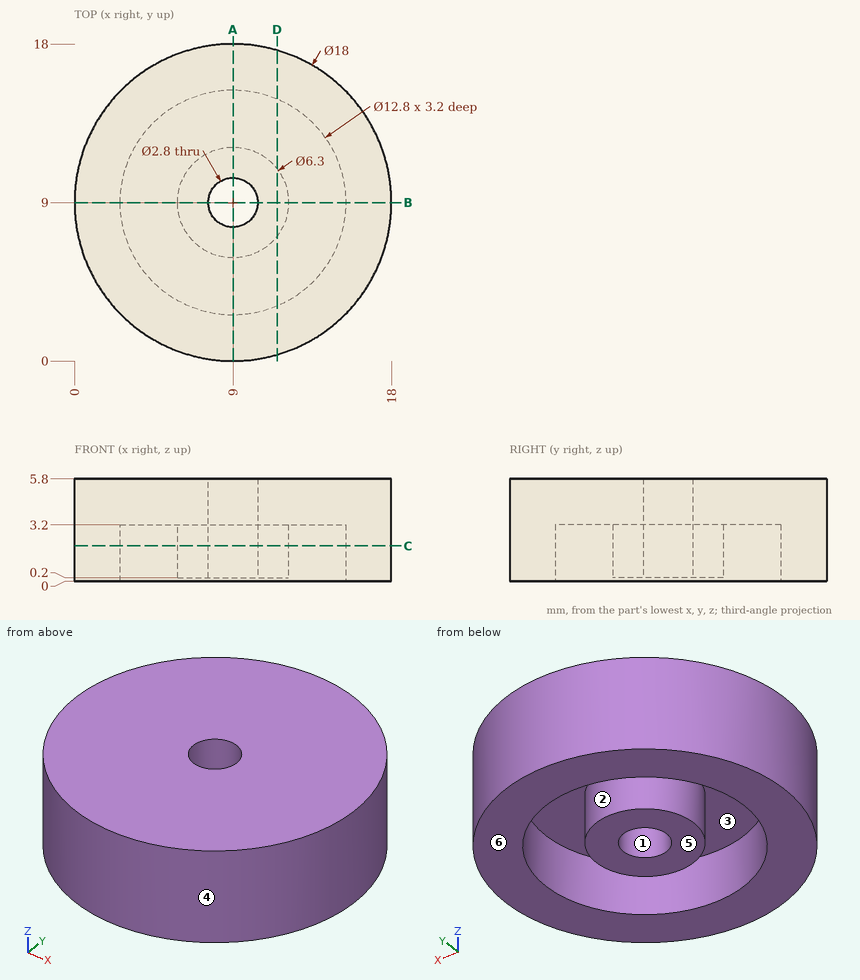
Design review of the part shown in the three views and the two pictorial views. Dimensions are in mm from the part's minimum x, y and z. A direction names the side the tool comes from. Round coordinates to 2 decimals unless told otherwise and drop trailing zeros. Write each loop counter-clockwise with the first axis right and the second up, starting at its lowest first coordinate (ties: lowest second). Pieces come first, ordered by that corner, then holes.
Item 1: Wall thickness on L1, parallel to Y at x = 9, z = 2.6; L2, parallel to X at y = 9.5, z = 1.3; L3, parallel to Y at x = 9, z = 4.1: over which ranges is each line inside the solid? List them lowest first.
Item 2: Consider section A-A on x = 9. Give the boundary of the cut face in (y, z).
Item 3: For pin 1 Ø2.5 at (x, y) = (9, 9) entering from +Z (3 decimals); pin 2 Ø2 at (x, z) = (13.5, 3.5) entering from +Y; pin 3 Ø5 at (x, y) = (9.5, 8) entering from -Z; pin 4 Ø1.5 at (x, y) = (2, 13.5) entering from -Z, all flat-tipped, find the tip position at first contact; note any pin that passes through.
Item 4: Consider section C-C on z = 2. Give the boundary of the cut face in (x, y).
Item 5: Consider section D-D on x = 11.5. Give the boundary of the cut face in (y, z), and give its area (3 significant figures).
Item 6: For the marked faces 1 and 2, list the 3-axis set-ups (+Z, -Z, +X, -X, +Y, -Y) from which the entire face can be reached by the end or side of a thin tool; tool diameter is ignored.
Item 7: Draft analysis for pull direction X (two halves, no side actions). For the marked faces 3, 4, 5 and 6, state which applies: released by +X, released by -X, zero draft, split by the parting line, or undercut.
Check values:
1. L1: y = 0 to 2.6, 5.85 to 7.6, 10.4 to 12.15, 15.4 to 18
1. L2: x = 0.01 to 2.62, 5.89 to 7.69, 10.31 to 12.11, 15.38 to 17.99
1. L3: y = 0 to 7.6, 10.4 to 18
2. outline: (0, 0) - (2.6, 0) - (2.6, 3.2) - (5.85, 3.2) - (5.85, 0.2) - (7.6, 0.2) - (7.6, 5.8) - (0, 5.8) - close; (10.4, 0.2) - (12.15, 0.2) - (12.15, 3.2) - (15.4, 3.2) - (15.4, 0) - (18, 0) - (18, 5.8) - (10.4, 5.8) - close
3. pin 1: passes through
3. pin 2: stops at y = 17.29
3. pin 3: stops at z = 0.2
3. pin 4: stops at z = 0
4. outline: circle Ø18 at (9, 9); circle Ø6.3 at (9, 9); hole circle Ø12.8 at (9, 9); hole circle Ø2.8 at (9, 9)
5. outline: (0.35, 0) - (3.11, 0) - (3.11, 3.2) - (7.08, 3.2) - (7.08, 0.2) - (10.92, 0.2) - (10.92, 3.2) - (14.89, 3.2) - (14.89, 0) - (17.65, 0) - (17.65, 5.8) - (0.35, 5.8) - close
5. area: 74.1 mm2
6. face 1: +Z, -Z
6. face 2: -Z
7. face 3: undercut
7. face 4: split by the parting line
7. face 5: undercut
7. face 6: zero draft
